Autodesk Inventor part; units mm, degrees
ref_plane "YZ Plane" through (0, 0, 0) normal (1, 0, 0) x (0, 1, 0)
ref_plane "XZ Plane" through (0, 0, 0) normal (0, 1, 0) x (-1, 0, 0)
ref_plane "XY Plane" through (0, 0, 0) normal (0, 0, 1) x (1, 0, 0)
sketch "Sketch1" plane through (0, 0, 0) normal (1, 0, 0) x (0, 1, 0)
  line L0 (0, 0) -> (0, -20)
  line L1 (0, 0) -> (3.975, 0)
  line L2 (3.975, 0) -> (3.975, -7)
  line L3 (3.975, -7) -> (5.95, -9.25)
  line L4 (5.95, -9.25) -> (5.95, -10.75)
  line L5 (5.95, -10.75) -> (3.975, -13)
  line L6 (3.975, -13) -> (3.975, -20)
  line L7 (3.975, -20) -> (0, -20)
  dimension "d0" = 7.95
  dimension "d1" = 20
  dimension "d2" = 6
  dimension "d3" = 1.5
  dimension "d4" = 11.9
revolve "Revolution1" add sketch "Sketch1" angle 360 about axis through (0, 0, 0) along (0, 0, -1)
fillet "Fillet1" radius 0.5 2 edges at (0, -3.975, 0) (0, -3.975, -20)
properties part number "RailPlug" material "ABS Plastic"
Model file for the job. Use its own axes, mm. A direction names the side the tool comes from. Give positions to 0.01 mm unless a question says otherwise; leave off trailing zeros. Order: outer loops, then holes, each group sorted by start corner. A loop starts at its lowest first (then second) coordinate and runs counter-clockwise, first axis right, second up. Notation, with made-up numbers: M -28.5,76 L 9.5,76 A23 cw 9.5,107 Z; hole C 11,47.25 d4. An arc over 180 degrees is marked long. Write item = value, one per line.
Q1. Cut at A-A, the plane x = 0. List the corners of the cut face in (y, z) (3 decimals), then the cut area to 3 significant figures.
Derived:
outline = M -5.95,-10.75 L -3.975,-13 L -3.975,-19.5 A0.5 ccw -3.475,-20 L 3.475,-20 A0.5 ccw 3.975,-19.5 L 3.975,-13 L 5.95,-10.75 L 5.95,-9.25 L 3.975,-7 L 3.975,-0.5 A0.5 ccw 3.475,0 L -3.475,0 A0.5 ccw -3.975,-0.5 L -3.975,-7 L -5.95,-9.25 Z
area = 174 mm2
Q2. Tool access for faces 1 (the flat face through (0, 0, -20)), 2 (the cylindrical face through (-3.88, -0.86, -3.8)), 3 (the cylindrical face through (-3.88, -0.86, -16.3)): list every direction of +Z, -Z, +X, -X, +Y, -Y with a clear straight run to the whole face (end or side of a thin tool).
Derived:
face_1 = -Z, +X, -X, +Y, -Y
face_2 = +Z
face_3 = -Z
Q3. Drill centre lines: line 1 (X direction, y = -4.75, z = -9); line 2 (Y direction, x = -1.5, z = -2.25); line 3 (Y direction, x = 0.5, z = -4.5). Where is each one in solid material? Low to high. Write a range as [from, to].
Derived:
line_1 = [-3.21, 3.21]
line_2 = [-3.68, 3.68]
line_3 = [-3.94, 3.94]
Q4. Cut at C-C, the plane z = -4.25. List the corners of the cut face in (x, y) (3 decimals), then the cut area to 3 significant figures.
Derived:
outline = C 0,0 d7.95
area = 49.6 mm2
Q5. Flat gauge pins, fed straight in: pin 1 (6 mm diameter, centred on x = -1.5, z = -10, fed in from +Y); pin 2 (4 mm diameter, centred on x = -2, z = -7.5, fed in from +Y); pin 3 (1.5 mm diameter, centred on x = 1.5, z = -4, fed in from +Y); pin 4 (5 mm diameter, centred on y = -3.5, z = -13.5, fed in from -X). Where does each tip first touch, or does it go through?
Derived:
pin_1 = 5.95
pin_2 = 5.86
pin_3 = 3.9
pin_4 = -4.96
